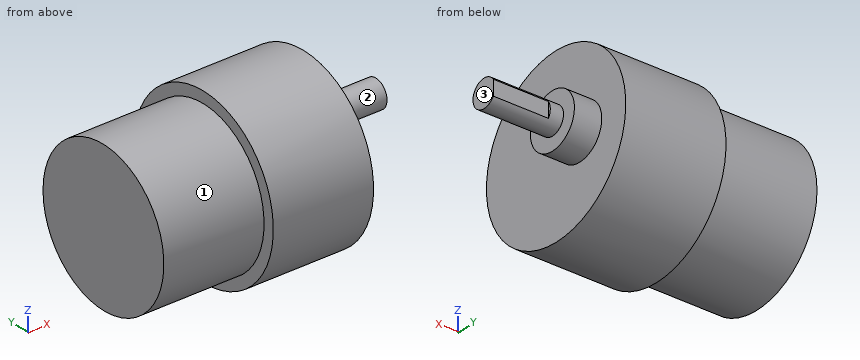
Autodesk Inventor part; units mm, degrees
ref_plane "YZ Plane" through (0, 0, 0) normal (1, 0, 0) x (0, 1, 0)
ref_plane "XZ Plane" through (0, 0, 0) normal (0, 1, 0) x (-1, 0, 0)
ref_plane "XY Plane" through (0, 0, 0) normal (0, 0, 1) x (1, 0, 0)
sketch "Sketch1" plane through (0, 0, 0) normal (1, 0, 0) x (0, 1, 0)
  circle A0 centre (0, 0) radius 16.35
  dimension "d0" = 32.7
extrude "Extrusion1" add sketch "Sketch1" along normal blind 22
sketch "Sketch2" plane through (22, 0, 0) normal (1, 0, 0) x (0, 0, -1)
  circle A0 centre (0, 0) radius 18.85
  dimension "d3" = 37.7
extrude "Extrusion2" add sketch "Sketch2" along normal blind 22
sketch "Sketch3" plane through (44, 0, 0) normal (1, 0, 0) x (0, 0, -1)
  circle A0 centre (0, 6.4) radius 5.95
  circle A1 centre (0, 0) radius 18.85
  line L0 (0, 18.85) -> (0, 12.35) construction
  dimension "d8" = 11.9
  dimension "d7" = 6.5
extrude "Extrusion3" add sketch "Sketch3" along normal blind 6 contours A0
sketch "Sketch4" plane through (50, 6.4, 0) normal (1, 0, 0) x (0, 0, -1)
  circle A0 centre (0, 0) radius 5.95
  circle A1 centre (0, 0) radius 3
  point P0 (0, -6.4)
  dimension "d14" = 6
extrude "Extrusion4" add sketch "Sketch4" along normal blind 15 contours A1
sketch "Sketch5" plane through (65, 6.4, 0) normal (1, 0, 0) x (0, 0, -1)
  circle A0 centre (0, 0) radius 3
  line L0 (-1.6583, 2.5) -> (1.6583, 2.5)
  point P0 (0, 2.5)
  dimension "d17" = 2.5
extrude "Extrusion5" cut sketch "Sketch5" against normal blind 12.1 contours L0 A0 picked at (-0.1169, 2.6598)
properties part number "Drive Motor approximate"
Source: CAD feature listing. Evaluate the final solid. Frame: model axes, mm. Face numbers are marked on the shaded views. A direction names the side the tool comes from. Coordinates: 2 decimals unless noted, no trailing zeros. Write each loop counter-clockwise with the first axis right and the second up, starting at its lowest first coordinate (ties: lowest second). Pieces come first, ordered by that corner, then holes. Notation, with made-up numbers: (-16, 63) -> (13, 63) arc R15 cw to (13, 76) -> close; hole circle Ø7 at (3.5, -28.5). An arc over 180 degrees is marked (long way). Return JSON: item names as keys, results as strings. Group by question number.
1) Section query A-A, the plane z = 0. Return loops of the section in (x, y).
2) Section query D-D, the plane z = -15.5. Return loops of the section in (x, y), plus the area to 3 significant figures.
3) Section query C-C, the plane x = 16.5. Return loops of the section in (y, z), plus the area to 3 significant figures.
4) Section query B-B, the plane y = -2.5. Return loops of the section in (x, z).
5) Ray query, line 1 along X through (y, z) = (14.5, -6); line 2 along X through (y, z) = (-14, -8.5); line 3 along Z through (x, y) = (35.5, 7). Return the intervals inside material, ascending.
6) Contact query for flat-ended pins moving along their axis: P1, Ø5, axis at y = 3, z = 13.5, coming from the +X side; P2, Ø2, axis at x = 31.5, y = -2, coming from the -Z side; P3, Ø6, axis at x = 48, y = -1.5, coming from the +Z side. Output: stop coordinate, or through.
7) Set-up query: the marked faces 1, 2 and 3. Return all of +Z, -Z, +X, -X, +Y, -Y with unobstructed straight access to the full face (end or side cutting, diameter ignored); none if empty.
From the geometry:
{
 "1": {"outline": "(0, -16.35) -> (22, -16.35) -> (22, -18.85) -> (44, -18.85) -> (44, 0.45) -> (50, 0.45) -> (50, 3.4) -> (65, 3.4) -> (65, 8.9) -> (52.9, 8.9) -> (52.9, 9.4) -> (50, 9.4) -> (50, 12.35) -> (44, 12.35) -> (44, 18.85) -> (22, 18.85) -> (22, 16.35) -> (0, 16.35) -> close"},
 "2": {"outline": "(0, -5.2) -> (22, -5.2) -> (22, -10.73) -> (44, -10.73) -> (44, 10.73) -> (22, 10.73) -> (22, 5.2) -> (0, 5.2) -> close", "area": "701 mm²"},
 "3": {"outline": "circle Ø32.7 at (0, 0)", "area": "840 mm²"},
 "4": {"outline": "(0, -16.16) -> (22, -16.16) -> (22, -18.68) -> (44, -18.68) -> (44, 18.68) -> (22, 18.68) -> (22, 16.16) -> (0, 16.16) -> close"},
 "5": {"line 1": "0 to 44", "line 2": "22 to 44", "line 3": "-17.5 to 17.5"},
 "6": {"P1": "x = 44", "P2": "z = -18.82", "P3": "z = 3.38"},
 "7": {"face 1": "-X", "face 2": "+X", "face 3": "+Z, -Z, +X, +Y, -Y"}
}
